from build123d import *

# Parameters (mm, degrees)
PAD006_DEPTH           = 32
SKETCH014_R            = 6
POCKET004_DEPTH        = 232.77922
LINEARPATTERN002_COUNT = 4
LINEARPATTERN002_PITCH = 130


with BuildPart() as part:
    # Sketch013 → Pad006 (new body)
    with BuildSketch(Plane.XY):
        Polygon((-385.11428, 291.5), (10.26148, 14.654912), (6.820021, 9.74), (-388.555739, 286.585088), align=None)
    extrude(amount=PAD006_DEPTH)

    # Sketch014 (on Face3 of Pad006) → Pocket004 (cut, through all)
    with BuildSketch(Plane(origin=(6.820021, 9.74, 0), x_dir=(0.819152, -0.573576, 0), z_dir=(-0.573576, -0.819152, 0))):
        with Locations((-462.664681, 16)):
            Circle(SKETCH014_R)
    pocket004 = extrude(amount=-POCKET004_DEPTH, mode=Mode.SUBTRACT)

    # LinearPattern002: Pocket004 ×4
    with Locations(*[Vector(0.819152, -0.573576, 0) * (i * LINEARPATTERN002_PITCH) for i in range(1, LINEARPATTERN002_COUNT)]):
        add(pocket004, mode=Mode.SUBTRACT)


with BuildPart() as part_1:
    # Body005 placement: moved
    add(part.part.moved(Location((0, 0, 9))))


solid = part_1.part
Work out the finished part from the listing and answer in its coordinate system (mm). Coordinates: 2 decimals unless noted, no trailing zeros. Write each loop counter-clockwise with the first axis right and the second up, starting at its lowest first coordinate (ties: lowest second). Pieces come first, ordered by that corner, then holes.
1. The part is cut by section B-B, the plane x = -146. Write down the section's boundary in (y, z).
Results list:
outline: (116.75, 9) - (124.07, 9) - (124.07, 41) - (116.75, 41) - close
2. Consider line 1 along X through (y, z) = (21, 19); line 2 along Y through (x, z) = (-344.5, 36); line 3 along Y through (x, z) = (-347, 29.5). Determine where each line is inside the solid, lowest interval first.
Results list:
line 1: x = -9.26 to 1.2
line 2: y = 255.74 to 263.06
line 3: y = 257.49 to 264.81
3. Flat-ended cylindrical pins translate along their axes: pin 1 (12 mm diameter, centred on y = 49, z = 28, fed in from +X); pin 2 (12 mm diameter, centred on x = -257.5, z = 22.5, fed in from +Y); pin 3 (1.5 mm diameter, centred on x = -256, z = 13, fed in from +Y). Find the tip coordinate at first contact, or state that the pin passes through.
Results list:
pin 1: stops at x = -30.22
pin 2: stops at y = 205.56
pin 3: stops at y = 201.62
4. The part is cut by section A-A, the plane z = 36. Write down the section's boundary in (x, y), and give its area (3 significant figures).
Results list:
outline: (-388.56, 286.59) - (6.82, 9.74) - (10.26, 14.65) - (-385.11, 291.5) - close
area: 2,900 mm2
5. For a pull along Z with two mould halves and no side action, classify faces 1 (the flat face through (-188, 151, 41)), 2 (the cylindrical face through (-267.89, 205.7, 21.35)), 3 (the flat face through (-188.1, 146.225, 24.776)) as +Z half, -Z half, draft (parallel to the pull), parting line (faces both ways), or undercut.
Results list:
face 1: +Z half
face 2: undercut
face 3: draft
